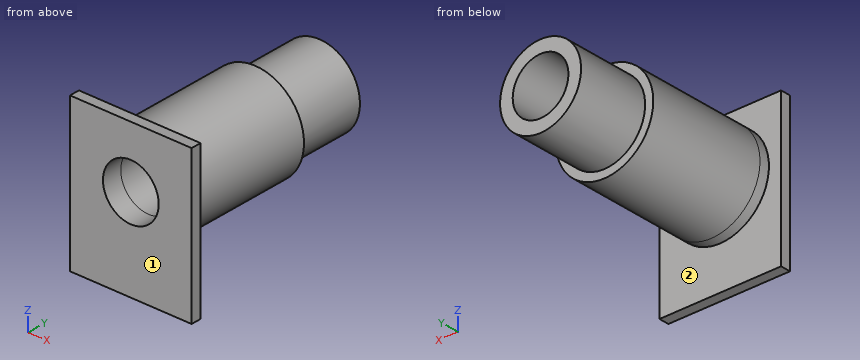
Autodesk Inventor part; units mm, degrees
ref_plane "YZ Plane" through (0, 0, 0) normal (1, 0, 0) x (0, 1, 0)
ref_plane "XZ Plane" through (0, 0, 0) normal (0, 1, 0) x (-1, 0, 0)
ref_plane "XY Plane" through (0, 0, 0) normal (0, 0, 1) x (1, 0, 0)
sketch "Sketch1" plane through (0, 0, 0) normal (0, 1, 0) x (-1, 0, 0)
  circle A0 centre (0, 0) radius 6.096
  circle A1 centre (0, 0) radius 3.4925
  dimension "d0" = 12.192
  dimension "d1" = 6.985
extrude "Extrusion1" add sketch "Sketch1" along normal blind 15.24
sketch "Sketch2" plane through (0, 15.24, 0) normal (0, 1, 0) x (1, 0, 0)
  circle A0 centre (0, 0) radius 3.4925
  circle A1 centre (0, 0) radius 6.096
  circle A2 centre (0, 0) radius 3.4925
  circle A3 centre (0, 0) radius 5.08
  dimension "d4" = 10.16
extrude "Extrusion2" add sketch "Sketch2" along normal blind 9.144 contours A3
sketch "Sketch3" plane through (0, 0, 0) normal (0, -1, 0) x (1, 0, 0)
  circle A0 centre (0, 0) radius 3.4925
  circle A1 centre (0, 0) radius 6.096
  circle A2 centre (0, 0) radius 3.4925
  circle A3 centre (0, 0) radius 6.096
extrude "Extrusion3" add sketch "Sketch3" along normal blind 2.54
sketch "Sketch4" plane through (0, -2.54, 0) normal (0, -1, 0) x (1, 0, 0)
  circle A0 centre (0, 0) radius 6.096
  circle A1 centre (0, 0) radius 6.096
  line L0 (-7.62, 7.62) -> (7.62, 7.62)
  line L1 (7.62, 7.62) -> (7.62, -11.43)
  line L2 (7.62, -11.43) -> (-7.62, -11.43)
  line L3 (-7.62, -11.43) -> (-7.62, 7.62)
  dimension "d12" = 15.24
  dimension "d13" = 19.05
  dimension "d14" = 7.62
  dimension "d15" = 7.62
extrude "Extrusion4" add sketch "Sketch4" against normal blind 1.27
properties part number "Tube_Part"
CAD build for the part. Positions are in the model's coordinates, mm. Face numbers are marked on the shaded views. A direction names the side the tool comes from. Round coordinates to 2 decimals unless told otherwise and drop trailing zeros. Write each loop counter-clockwise with the first axis right and the second up, starting at its lowest first coordinate (ties: lowest second). Pieces come first, ordered by that corner, then holes.
(1) Drop flat-ended pins along their axis: P1, Ø1, axis at x = 5.5, z = 4, coming from the +Y side; P2, Ø4, axis at y = 11, z = -7.5, coming from the -X side; P3, Ø1, axis at x = -4.5, y = 15.5, coming from the +Z side. Give the stop position or say it passes through.
(2) Probe line 1 along Z through (x, y) = (0, -2); line 2 along Z through (x, y) = (0, 10.5); line 3 along X through (y, z) = (-1.95, 0). List the from-to ranges inside material, lowest first.
(3) Slice it at D-D, the plane z = -10.25. Write the cut outline in (x, y).
(4) 3-axis set-ups, long thin cutter, end or side, ignore diameter. For the marked faces 1 and 2: which of +Z, -Z, +X, -X, +Y, -Y reach the whole face in a straight line?
(5) Slice it at B-B, the plane y = 10.75. Write the cut outline in (x, z) (1 decimal), and give its area (3 significant figures).
(6) Slice it at C-C, the plane z = -0.75. Write the cut outline in (x, y), and give its area (3 significant figures).
From the geometry:
1. P1: stops at y = -1.27
1. P2: stops at x = -2.63
1. P3: stops at z = 4.54
2. line 1: z = -11.43 to -3.49, 3.49 to 7.62
2. line 2: z = -6.1 to -3.49, 3.49 to 6.1
2. line 3: x = -7.62 to -3.49, 3.49 to 7.62
3. outline: (-7.62, -2.54) - (7.62, -2.54) - (7.62, -1.27) - (-7.62, -1.27) - close
4. face 1: +Z, -Z, +X, -X, -Y
4. face 2: +Y
5. outline: circle Ø12.2 at (0, 0); hole circle Ø7 at (0, 0)
5. area: 78.4 mm2
6. outline: (-7.62, -2.54) - (-3.41, -2.54) - (-3.41, 24.38) - (-5.02, 24.38) - (-5.02, 15.24) - (-6.05, 15.24) - (-6.05, -1.27) - (-7.62, -1.27) - close; (3.41, -2.54) - (7.62, -2.54) - (7.62, -1.27) - (6.05, -1.27) - (6.05, 15.24) - (5.02, 15.24) - (5.02, 24.38) - (3.41, 24.38) - close
6. area: 127 mm2
